```python
from build123d import *

# Parameters (mm, degrees)
SKETCH028_W             = 200
SKETCH028_H             = 140
PAD014_DEPTH            = 6
SKETCH026_W             = 179
SKETCH026_H             = 119
PAD015_DEPTH            = 11
SKETCH027_W             = 150.5
SKETCH027_H             = 100.5
POCKET012_DEPTH         = 2.5
SKETCH025_W             = 140.5
SKETCH025_H             = 90.5
POCKET011_DEPTH         = 12
BODY007_PLACEMENT_ANGLE = 180


with BuildPart() as part:
    # Sketch028 → Pad014 (new body)
    with BuildSketch(Plane.XY):
        with Locations((100, 70)):
            Rectangle(SKETCH028_W, SKETCH028_H)
    extrude(amount=PAD014_DEPTH)

    # Sketch026 → Pad015 (join)
    with BuildSketch(Plane.XY):
        with Locations((100, 70)):
            Rectangle(SKETCH026_W, SKETCH026_H)
    extrude(amount=PAD015_DEPTH)

    # Sketch027 → Pocket012 (cut)
    with BuildSketch(Plane.XY):
        with Locations((100, 70)):
            Rectangle(SKETCH027_W, SKETCH027_H)
    extrude(amount=POCKET012_DEPTH, mode=Mode.SUBTRACT)

    # Sketch025 → Pocket011 (cut)
    with BuildSketch(Plane.XY):
        with Locations((99.75, 70)):
            Rectangle(SKETCH025_W, SKETCH025_H)
    extrude(amount=POCKET011_DEPTH, mode=Mode.SUBTRACT)


with BuildPart() as part_1:
    # Body007 placement: moved
    add(part.part.moved(Location((175.5, -20, -0.5))).rotate(Axis((175.5, -20, -0.5), (0, 1, 0)), BODY007_PLACEMENT_ANGLE))


solid = part_1.part
```
Could you check a few things on this model? Use its own coordinates, in mm. A direction names the side the tool comes from. Round coordinates to 2 decimals unless told otherwise and drop trailing zeros. Loops run counter-clockwise (first coordinate to the right, second up) from the corner with the lowest first, then second, coordinate; pieces in that order, holes last. Notation, with made-up numbers: (51, 5) - (86, 5) arc R7 ccw to (86, 13) - close; hole circle Ø7 at (-19.75, 86). An arc over 180 degrees is marked (long way). Answer as CSV lines item,"result".
1. For pin 1 Ø2.5 at (y, z) = (65, -9.5) entering from -X; pin 2 Ø1.5 at (x, y) = (103, 1) entering from +Z; pin 3 Ø1.5 at (y, z) = (61, -10) entering from +X, each with a flat end and sliding along its axis, tell me the tip position at first contact or that it passes through.
Filled in:
pin 1,"stops at x = -14"
pin 2,"stops at z = -3"
pin 3,"stops at x = 165"
2. Please list where these lines run through material, in increasing order: line 1 along X through (y, z) = (21, -2.5); line 2 along X through (y, z) = (29, -4.5); line 3 along Y through (x, z) = (67, -1.5). Write a range as [from, to].
Filled in:
line 1,"x = [-24.5, 0.25], [150.75, 175.5]"
line 2,"x = [-24.5, 5.5], [146, 175.5]"
line 3,"y = [-20, -0.25], [100.25, 120]"
3. On a 3-axis mill with a long thin cutter (end or side, diameter ignored), from which of +Z, -Z, +X, -X, +Y, -Y can I reach the whole of each face in a straight line? I mean faces 5 (the face through (165, 49, -9)), 6 (the face through (77, 95.25, -7)), 7 (the face through (77, 109.5, -9)), 8 (the face through (-14, 49, -9)). Say none if no direction works.
Filled in:
face 5,"-Z, +X, +Y, -Y"
face 6,"+Z, -Z"
face 7,"-Z, +X, -X, +Y"
face 8,"-Z, -X, +Y, -Y"
4. I want a section at D-D on y = -6. List the corners of the cut face in (x, z) for me.
Filled in:
outline,"(-24.5, -6.5) - (-14, -6.5) - (-14, -11.5) - (165, -11.5) - (165, -6.5) - (175.5, -6.5) - (175.5, -0.5) - (-24.5, -0.5) - close"
5. We'd pull the mould along Y, two halves only. Please class faces 1 (the face through (81, 2, -3)), 2 (the face through (77, -9.5, -9)), 3 (the face through (-24.5, 49, -3)), 4 (the face through (77, 4.75, -7)): +Y half, -Y half, draft (parallel to the pull), parting line (faces both ways), or undercut.
Filled in:
face 1,"undercut"
face 2,"-Y half"
face 3,"draft"
face 4,"undercut"
6. I want a section at B-B on x = 35.5. List the corners of the cut face in (y, z) for me, then the cut area to 4 significant figures.
Filled in:
outline,"(-20, -6.5) - (-9.5, -6.5) - (-9.5, -11.5) - (4.75, -11.5) - (4.75, -3) - (-0.25, -3) - (-0.25, -0.5) - (-20, -0.5) - close; (95.25, -11.5) - (109.5, -11.5) - (109.5, -6.5) - (120, -6.5) - (120, -0.5) - (100.25, -0.5) - (100.25, -3) - (95.25, -3) - close"
area,"414.5 mm^2"
7. I want a section at A-A on y = 39.5. List the corners of the cut face in (x, z) for me, then the cut area to 4 significant figures.
Filled in:
outline,"(-24.5, -6.5) - (-14, -6.5) - (-14, -11.5) - (5.5, -11.5) - (5.5, -3) - (0.25, -3) - (0.25, -0.5) - (-24.5, -0.5) - close; (146, -11.5) - (165, -11.5) - (165, -6.5) - (175.5, -6.5) - (175.5, -0.5) - (150.75, -0.5) - (150.75, -3) - (146, -3) - close"
area,"524.5 mm^2"
8. I want a section at C-C on z = -9.25. List the corners of the cut face in (x, y) for me, then the cut area to 3 significant figures.
Filled in:
outline,"(-14, -9.5) - (165, -9.5) - (165, 109.5) - (-14, 109.5) - close; hole (5.5, 4.75) - (146, 4.75) - (146, 95.25) - (5.5, 95.25) - close"
area,"8,590 mm^2"
